```python
from build123d import *

# Parameters (mm, degrees)
BOSS_EXTRUDE1_DEPTH                                 = 40
FILLET1_R                                           = 20
CUT_EXTRUDE2_REACH                                  = 150.682
SKETCH3_R                                           = 12
SKETCH4_R                                           = 10
CUT_EXTRUDE3_DEPTH                                  = 7
CIRPATTERN1_COUNT                                   = 12
F_10_0_10_DIAMETER_HOLE1_D                          = 10
SKETCH8_R                                           = 8.5
CUT_EXTRUDE4_DEPTH                                  = 23
CBORE_FOR_M6_HEX_SOCKET_HEAD_CAP_SCREW1_D           = 6.4
CBORE_FOR_M6_HEX_SOCKET_HEAD_CAP_SCREW1_CBORE_D     = 11
CBORE_FOR_M6_HEX_SOCKET_HEAD_CAP_SCREW1_CBORE_DEPTH = 6.4
F_8_0MM_DOWEL_HOLE1_D                               = 8


with BuildPart() as part:
    # Sketch1 → Boss-Extrude1 (new body)
    with BuildSketch(Plane(origin=(0, 0, 0), x_dir=(1, 0, 0), z_dir=(0, 1, 0))):
        with BuildLine():
            Line((-90, 0), (-90, 39.504902432))
            ThreePointArc((-90, 39.504902432), (-85.182396525, 94.862332258), (-30.561841884, 84.652075111))
            ThreePointArc((-30.561841884, 84.652075111), (0, 90), (30.561841884, 84.652075111))
            ThreePointArc((30.561841884, 84.652075111), (85.182396525, 94.862332258), (90, 39.504902432))
            Line((90, 39.504902432), (90, 0))
            ThreePointArc((90, 0), (0, -90), (-90, 0))
        make_face()
    extrude(amount=-BOSS_EXTRUDE1_DEPTH)

    # Fillet1
    fillet1_edges = [part.edges().sort_by_distance(p)[0] for p in [
        (30.561841884, -20, -84.652075111),
        (90, -20, -39.504902432),
        (-90, -20, -39.504902432),
        (-30.561841884, -20, -84.652075111),
    ]]
    fillet(fillet1_edges, radius=FILLET1_R)

    # Sketch3 → Cut-Extrude2 (cut, up to next)
    with BuildSketch(Plane(origin=(0, 0, 0), x_dir=(1, 0, 0), z_dir=(0, 1, 0)), mode=Mode.PRIVATE) as cut_extrude2_sk1:
        with Locations(Location((-62.5, 65, 0), (0, 0, 270))):
            Circle(SKETCH3_R)
    cut_extrude2_tool1 = extrude(cut_extrude2_sk1.sketch, amount=-CUT_EXTRUDE2_REACH, mode=Mode.PRIVATE) & part.part
    # Sketch3 → Cut-Extrude2 (cut, up to next)
    with BuildSketch(Plane(origin=(0, 0, 0), x_dir=(1, 0, 0), z_dir=(0, 1, 0)), mode=Mode.PRIVATE) as cut_extrude2_sk2:
        with Locations(Location((62.5, 65, 0), (0, 0, 270))):
            Circle(SKETCH3_R)
    cut_extrude2_tool2 = extrude(cut_extrude2_sk2.sketch, amount=-CUT_EXTRUDE2_REACH, mode=Mode.PRIVATE) & part.part
    add(cut_extrude2_tool1.solids().sort_by_distance((-62.5, 0, -65))[0], mode=Mode.SUBTRACT)
    add(cut_extrude2_tool2.solids().sort_by_distance((62.5, 0, -65))[0], mode=Mode.SUBTRACT)

    # Sketch4 → Cut-Extrude3 (cut)
    with BuildSketch(Plane(origin=(0, 0, 0), x_dir=(1, 0, 0), z_dir=(0, 1, 0))):
        with Locations(Location((0, 45, 0), (0, 0, 270))):
            Circle(SKETCH4_R)
    cut_extrude3 = extrude(amount=-CUT_EXTRUDE3_DEPTH, mode=Mode.SUBTRACT)

    # CirPattern1: Cut-Extrude3 ×12 about axis
    cirpattern1_axis = Axis((0, 0, 0), (0, 1, 0))
    for i in range(1, CIRPATTERN1_COUNT):
        add(cut_extrude3.rotate(cirpattern1_axis, i * 360 / CIRPATTERN1_COUNT), mode=Mode.SUBTRACT)

    # Ø10.0 (10) Diameter Hole1 (through all)
    with Locations(Plane(origin=(0, 0, 0), x_dir=(1, 0, 0), z_dir=(0, 1, 0))):
        with Locations((0, 45), (45, 0), (0, -45), (-45, 0)):
            Hole(F_10_0_10_DIAMETER_HOLE1_D / 2)

    # Sketch8 → Cut-Extrude4 (cut)
    with BuildSketch(Plane.XZ.offset(40)):
        with Locations(Location((0, 45, 0), (0, 0, 270))):
            Circle(SKETCH8_R)
        with Locations(Location((45, 0, 0), (0, 0, 270))):
            Circle(SKETCH8_R)
        with Locations(Location((0, -45, 0), (0, 0, 270))):
            Circle(SKETCH8_R)
        with Locations(Location((-45, 0, 0), (0, 0, 270))):
            Circle(SKETCH8_R)
    extrude(amount=-CUT_EXTRUDE4_DEPTH, mode=Mode.SUBTRACT)

    # CBORE for M6 Hex Socket Head Cap Screw1 (through all)
    with Locations(Plane(origin=(0, -40, 0), x_dir=(-1, 0, 0), z_dir=(0, -1, 0))):
        with Locations((0, 22.5), (-19.485571585, -11.25), (19.485571585, -11.25)):
            CounterBoreHole(CBORE_FOR_M6_HEX_SOCKET_HEAD_CAP_SCREW1_D / 2, CBORE_FOR_M6_HEX_SOCKET_HEAD_CAP_SCREW1_CBORE_D / 2, CBORE_FOR_M6_HEX_SOCKET_HEAD_CAP_SCREW1_CBORE_DEPTH)

    # Ø8.0mm Dowel Hole1 (through all)
    with Locations(Plane(origin=(0, 0, 0), x_dir=(1, 0, 0), z_dir=(0, 1, 0))):
        with Locations((-22.5, 0), (22.5, 0)):
            Hole(F_8_0MM_DOWEL_HOLE1_D / 2)


solid = part.part
```
Model file for the job. Use its own axes, mm. A direction names the side the tool comes from. Give positions to 0.01 mm unless a question says otherwise; leave off trailing zeros. Loops run counter-clockwise (first coordinate to the right, second up) from the corner with the lowest first, then second, coordinate; pieces in that order, holes last. Notation, with made-up numbers: (-25.75, 16.5) -> (21.25, 16.5) arc R5 ccw to (21.25, 20.5) -> close; hole circle Ø9 at (86, -8.75). An arc over 180 degrees is marked (long way). Use CSV: the item, a comma, the result in double quotes. Start each with the question number.
1) Mould opens along Z. For faces 1 (the flat face through (-22, -7, -39)), 2 (the cylindrical face through (0, -20, -90)), 3 (the flat face through (-49, -17, -4)), 4 (the flat face through (-90, -20, -16)) say: released by +Z, released by -Z, zero draft, split by the parting line, or undercut.
2) Slice it at B-B on x = 62.5. Give the cut face in (y, z), plus the area to 3 significant figures.
3) Tool access for faces 5 (the cylindrical face through (-0.417, -16.565, -25.673)), 6 (the cylindrical face through (32.04, -3.45, 35.97)), 7 (the flat face through (90, -20, -17)): list every direction of +Z, -Z, +X, -X, +Y, -Y with a clear straight run to the whole face (end or side of a thin tool).
4) Slice it at D-D on x = 0. Give the number of separate pieces and of enclosed holes in the cut face, plus the area to 3 significant figures.
5) Wall check: line 1 (X direction, y = -9, z = -65); line 2 (Z direction, x = 52, y = -6); line 3 (X direction, y = -5, z = 22). Give the ranges that are in metal, low to high.
6) Flat gauge pins, fed straight in: pin 1 Ø18 at (x, z) = (38.97, 22.5) entering from +Y; pin 2 Ø1 at (x, y) = (-49, -19.5) entering from +Z; pin 3 Ø12 at (y, z) = (-22.5, -38) entering from -X; pin 4 Ø6 at (x, z) = (-44.5, 0.5) entering from +Y. Where does each tip first touch, or does it go through?
7) Slice it at A-A on z = -22.5. Give the cut face in (x, y).
8) Slice it at C-C on z = -65. Give the cut face in (x, y).
Computed values:
1,face 1,"undercut"
1,face 2,"released by -Z"
1,face 3,"undercut"
1,face 4,"zero draft"
2,outline,"(-40, -102.5) -> (0, -102.5) -> (0, -77) -> (-40, -77) -> close; (-40, -53) -> (0, -53) -> (0, 64.76) -> (-40, 64.76) -> close"
2,area,"5,730 mm^2"
3,face 5,"+Y, -Y"
3,face 6,"+Y"
3,face 7,"+Z, +X, +Y, -Y"
4,separate pieces,"4"
4,enclosed holes,"0"
4,area,"5,650 mm^2"
5,line 1,"x = -100 to -74.5, -50.5 to 50.5, 74.5 to 100"
5,line 2,"z = -101 to -70.81, -59.19 to -7.14, 7.14 to 73.46"
5,line 3,"x = -87.27 to -48.96, -28.98 to 28.98, 48.96 to 87.27"
6,pin 1,"stops at y = -7"
6,pin 2,"stops at z = 75.81"
6,pin 3,"stops at x = -93.57"
6,pin 4,"passes through"
7,outline,"(-90, -40) -> (-5.5, -40) -> (-5.5, -33.6) -> (-3.2, -33.6) -> (-3.2, 0) -> (-28.97, 0) -> (-28.97, -7) -> (-48.97, -7) -> (-48.97, 0) -> (-90, 0) -> close; (3.2, -33.6) -> (5.5, -33.6) -> (5.5, -40) -> (90, -40) -> (90, 0) -> (48.97, 0) -> (48.97, -7) -> (28.97, -7) -> (28.97, 0) -> (3.2, 0) -> close"
8,outline,"(-100, -40) -> (-74.5, -40) -> (-74.5, 0) -> (-100, 0) -> close; (-50.5, -40) -> (50.5, -40) -> (50.5, 0) -> (-50.5, 0) -> close; (74.5, -40) -> (100, -40) -> (100, 0) -> (74.5, 0) -> close"
